Geometry check sheet. Reference: drawing and pictorial views, mm from the part's lowest x, y, z. Round coordinates to 2 decimals unless told otherwise and drop trailing zeros. Order: outer loops, then holes, each group sorted by start corner. A loop starts at its lowest first (then second) coordinate and runs counter-clockwise, first axis right, second up. Notation, with made-up numbers: (-37, -39) -> (0, -39) arc R32 ccw to (0, -8) -> close; hole circle Ø6 at (37, 30.25). An arc over 180 degrees is marked (long way). Put each result on its own line as item: value.
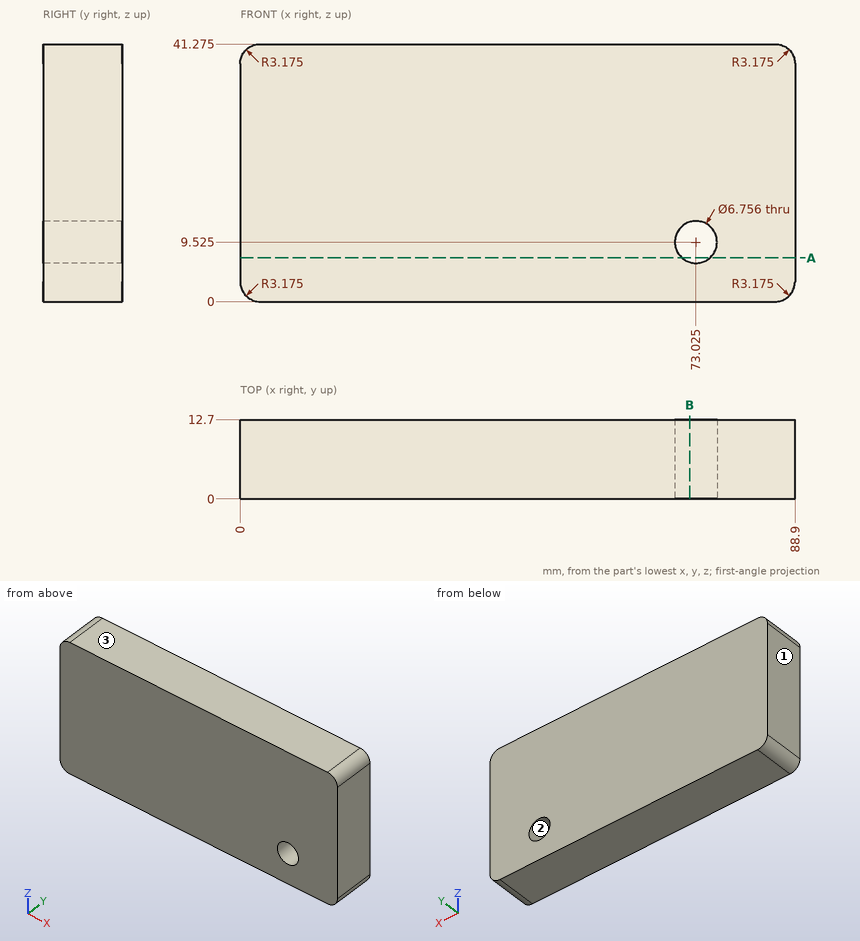
Item 1: Release check for a two-part mould opening along X. For the marked faces 1, 2 and 3 record: pulls with the +X half, pulls with the -X half, needs draft (parallel to the pull), parting line crosses it, or undercut.
Geometry check:
face 1: pulls with the -X half
face 2: undercut
face 3: needs draft
Item 2: Sectioned sample at B-B, the plane x = 72. Record the boundary of the cut face in (y, z) (1 decimal).
Geometry check:
outline: (0, 0) -> (12.7, 0) -> (12.7, 6.3) -> (0, 6.3) -> close; (0, 12.7) -> (12.7, 12.7) -> (12.7, 41.3) -> (0, 41.3) -> close
Item 3: Sectioned sample at A-A, the plane z = 7. Record the boundary of the cut face in (x, y), then the cut area to 3 significant figures.
Geometry check:
outline: (0, 0) -> (70.78, 0) -> (70.78, 12.7) -> (0, 12.7) -> close; (75.27, 0) -> (88.9, 0) -> (88.9, 12.7) -> (75.27, 12.7) -> close
area: 1,070 mm2
Item 4: Material ranges on line 1 along X through (y, z) = (2.75, 7); line 2 along X through (y, z) = (6, 9.5); line 3 along X through (y, z) = (4, 39), recorded low to high.
Geometry check:
line 1: 0 to 70.78, 75.27 to 88.9
line 2: 0 to 69.65, 76.4 to 88.9
line 3: 0.13 to 88.77
